Autodesk Inventor part; units mm, degrees
ref_plane "YZ Plane" through (0, 0, 0) normal (1, 0, 0) x (0, 1, 0)
ref_plane "XZ Plane" through (0, 0, 0) normal (0, 1, 0) x (-1, 0, 0)
ref_plane "XY Plane" through (0, 0, 0) normal (0, 0, 1) x (1, 0, 0)
sketch "Sketch1" plane through (0, 0, 0) normal (0, 0, 1) x (1, 0, 0)
  circle A0 centre (0, 0) radius 6.0688
extrude "Extrusion1" add sketch "Sketch1" along normal blind 101.6
sketch "Sketch2" plane through (0, 0, 101.6) normal (0, 0, 1) x (1, 0, 0)
  line L0 (-6.0688, 6.0688) -> (6.0688, 6.0688)
  line L1 (6.0688, 6.0688) -> (6.0688, -6.0688)
  line L2 (6.0688, -6.0688) -> (-6.0688, -6.0688)
  line L3 (-6.0688, -6.0688) -> (-6.0688, 6.0688)
extrude "Extrusion2" add sketch "Sketch2" along normal blind 12.7
sketch "Sketch3" plane through (6.0688, -6.0688, 101.6) normal (1, 0, 0) x (0, 0, -1)
  line L0 (-12.7, 12.1376) -> (-12.7, 0)
  circle A0 centre (-12.7, 6.0688) radius 3.175
  point P0 (101.6, 6.0688)
  dimension "d4" = 6.35
extrude "Extrusion3" cut sketch "Sketch3" against normal blind 12.7
sketch "Sketch4" plane through (6.0688, -6.0688, 101.6) normal (1, 0, 0) x (0, 0, -1)
  arc A0 (-12.7, 2.8938) -> (-12.7, 9.2438) centre (-12.7, 6.0688) ccw
  circle A1 centre (-12.7, 6.0688) radius 3.175
  circle A2 centre (-12.7, 6.0688) radius 6.0688
  point P0 (101.6, 6.0688)
extrude "Extrusion4" add sketch "Sketch4" against normal blind 12.7
sketch "Sketch5" plane through (-6.0688, 0, 101.6) normal (-1, 0, 0) x (0, 0, 1)
  arc A0 (12.7, 6.0688) -> (12.7, -6.0688) centre (12.7, 0) ccw
  line L0 (0, 6.0688) -> (12.7, 6.0688)
  line L1 (0, 0) -> (0, 6.0688)
  line L2 (0, -6.0688) -> (0, 0)
  line L3 (0, -6.0688) -> (12.7, -6.0688)
  line L4 (0, 6.0688) -> (38.3978, 6.0688)
  line L5 (38.3978, 6.0688) -> (38.3978, -6.0688)
  line L6 (38.3978, -6.0688) -> (0, -6.0688)
  line L7 (0, -6.0688) -> (0, 6.0688)
  point P0 (-101.6, 0)
extrude "Extrusion5" cut sketch "Sketch5" along normal blind 12.7 contours L4 L5 L6 A0
sketch "Sketch6" plane through (0, 0, 0) normal (0, 0, -1) x (-1, 0, 0)
  circle A0 centre (0, 0) radius 6.0688
  line L0 (0, 0) -> (0, 3.175)
  line L1 (0, 3.175) -> (-3.175, 3.175)
  line L2 (-3.175, 3.175) -> (3.175, 3.175)
  line L3 (3.175, 3.175) -> (3.175, -3.175)
  line L4 (3.175, -3.175) -> (-3.175, -3.175)
  line L5 (-3.175, -3.175) -> (-3.175, 3.175)
  dimension "d11" = 3.175
  dimension "d12" = 3.175
  dimension "d13" = 6.35
  dimension "d14" = 6.35
extrude "Extrusion6" add sketch "Sketch6" along normal blind 12.7 contours L2 L3 L4 L5 L1
fillet "Fillet1" radius 3.175 6 edges at (6.0688, 6.0688, 107.95) (6.0688, 0, 120.3688) (6.0688, -6.0688, 107.95) (-6.0688, 6.0688, 107.95) (-6.0688, 0, 120.3688) (-6.0688, -6.0688, 107.95)
sketch "Sketch7" plane through (0, 0, 0) normal (0, 0, -1) x (-1, 0, 0)
  circle A0 centre (0, 0) radius 6.0688
  circle A1 centre (0, 0) radius 9.906
  dimension "d18" = 19.812
extrude "Extrusion7" add sketch "Sketch7" against normal blind 101.6
sketch "Sketch8" plane through (0, 0, 101.6) normal (0, 0, 1) x (1, 0, 0)
  circle A0 centre (0, 0) radius 9.906
extrude "Extrusion8" cut sketch "Sketch8" along normal blind 101.6
sketch "Sketch9" plane through (0, 0, 101.6) normal (0, 0, 1) x (1, 0, 0)
  circle A0 centre (0, 0) radius 9.906
  circle A1 centre (0, 0) radius 6.35
  line L0 (-6.35, 6.35) -> (6.35, 6.35)
  line L1 (6.35, 6.35) -> (6.35, -6.35)
  line L2 (6.35, -6.35) -> (-6.35, -6.35)
  line L3 (-6.35, -6.35) -> (-6.35, 6.35)
  dimension "d23" = 12.7
extrude "Extrusion9" add sketch "Sketch9" along normal blind 12.7 contours A1 | L1 L2 A1 | A1 L0 L1 | A1 L3 L0 | L2 L3 A1
sketch "Sketch10" plane through (6.35, -6.35, 101.6) normal (1, 0, 0) x (0, 0, -1)
  line L0 (-12.7, 12.7) -> (-12.7, 0)
  circle A0 centre (-12.7, 6.35) radius 3.175
  point P0 (101.6, 6.35)
  dimension "d26" = 6.35
extrude "Extrusion10" cut sketch "Sketch10" against normal blind 12.7
sketch "Sketch11" plane through (6.35, -6.35, 101.6) normal (1, 0, 0) x (0, 0, -1)
  arc A0 (-12.7, 3.175) -> (-12.7, 9.525) centre (-12.7, 6.35) ccw
  circle A1 centre (-12.7, 6.35) radius 3.175
  circle A2 centre (-12.7, 6.35) radius 6.35
  point P0 (101.6, 6.35)
extrude "Extrusion11" add sketch "Sketch11" against normal blind 12.7
fillet "Fillet2" radius 3.175 6 edges at (6.35, 6.35, 107.95) (6.35, 0, 120.65) (6.35, -6.35, 107.95) (-6.35, 6.35, 107.95) (-6.35, 0, 120.65) (-6.35, -6.35, 107.95)
sketch "Sketch12" plane through (0, 0, -12.7) normal (0, 0, -1) x (-1, 0, 0)
  line L0 (3.175, 3.175) -> (3.175, -3.175)
  line L1 (-3.175, 3.175) -> (3.175, 3.175)
  line L2 (-3.175, -3.175) -> (-3.175, 3.175)
  line L3 (3.175, -3.175) -> (-3.175, -3.175)
  point P0 (0, 0)
extrude "Extrusion12" cut sketch "Sketch12" against normal blind 12.7
sketch "Sketch13" plane through (0, 0, 0) normal (0, 0, -1) x (-1, 0, 0)
  circle A0 centre (0, 0) radius 9.906
extrude "Extrusion13" add sketch "Sketch13" along normal blind 203.2
properties part number "linac arm12in"
Here's how the part is built. I have some questions about the finished solid (model axes, mm). A direction names the side the tool comes from. Coordinates: 2 decimals unless noted, no trailing zeros. Loops run counter-clockwise (first coordinate to the right, second up) from the corner with the lowest first, then second, coordinate; pieces in that order, holes last. Notation, with made-up numbers: (-0.75, 47) - (43.25, 47) arc R27 cw to (43.25, 74) - close; hole circle Ø7 at (57, 85). An arc over 180 degrees is marked (long way). Answer as CSV lines item,"result".
Q1. If we section it at B-B, the plane x = 0: Write out the boundary of the cut face in (y, z) (3 decimals), and give its area (3 significant figures).
Response:
outline,"(-9.906, -203.2) - (9.906, -203.2) - (9.906, 101.6) - (6.35, 101.6) - (6.35, 114.3) arc R6.35 ccw to (-6.35, 114.3) - (-6.35, 101.6) - (-9.906, 101.6) - close; hole circle Ø6.35 at (0, 114.3)"
area,"6,230 mm2"
Q2. For faces 4 (the face through (0, -6.35, 108)), 5 (the face through (0, 6.35, 108)), 6 (the face through (6.35, 0, 106)), 7 (the face through (-6.35, 0, 106)), which set-ups out of +Z, -Z, +X, -X, +Y, -Y let a thin tool reach every point of the face, with its end or its side?
Response:
face 4,"+Z, +X, -X, -Y"
face 5,"+Z, +X, -X, +Y"
face 6,"+Z, +X, +Y, -Y"
face 7,"+Z, -X, +Y, -Y"
Q3. We'd pull the mould along Z, two halves only. Please class faces 1 (the face through (0, 0, -203.2)), 2 (the face through (1.29, -9.82, -48.67)), 3 (the face through (0.09, -0.69, 111.2)): pulls with the +Z half, pulls with the -Z half, needs draft (parallel to the pull), parting line crosses it, or undercut.
Response:
face 1,"pulls with the -Z half"
face 2,"needs draft"
face 3,"undercut"
Q4. For pin 1 (4 mm diameter, centred on y = -5.5, z = -106, fed in from -X); pin 2 (5 mm diameter, centred on y = -6.5, z = 0.5, fed in from +X); pin 3 (1.5 mm diameter, centred on x = 6.5, z = -127.5, fed in from +Y), each with a flat end and sliding along its axis, tell me the tip position at first contact or that it passes through.
Response:
pin 1,"x = -9.27"
pin 2,"x = 9.06"
pin 3,"y = 8.07"
Q5. If I drill on L1, parallel to Y at x = -1.25, z = 114.3 (3 decimals); L2, parallel to Z at x = 2.5, y = 0 (3 decimals); L3, parallel to Z at x = 5.75, y = 5.25, over which ranges is the centre line in solid material (lowest first)? Write a range as [from, to].
Response:
L1,"[-6.35, -3.175], [3.175, 6.35]"
L2,"[-203.2, 111.125], [117.475, 120.65]"
L3,"[-203.2, 101.6]"
Q6. If we section it at C-C, the plane z = -89.5: Write out the boundary of the cut face in (x, y).
Response:
outline,"circle Ø19.81 at (0, 0)"
